```python
from build123d import *

# Parameters (mm, degrees)
SWEEP1_PROFILE_R = 0.425


with BuildPart() as part:
    # Sketch1 → Revolve1 (revolve)
    with BuildSketch(Plane(origin=(0, 0, 0), x_dir=(0, 0, -1), z_dir=(1, 0, 0)), mode=Mode.PRIVATE) as revolve1_sk:
        with BuildLine():
            Line((-2.775, -4.23083487), (-2.775, 0.55))
            Line((-2.775, 0.55), (-2.875, 0.55))
            Line((-2.875, 0.55), (-2.875, 1.55))
            Line((-2.875, 1.55), (-2.775, 1.55))
            Line((-2.775, 1.55), (-2.775, 3.55))
            Line((-2.775, 3.55), (-2.875, 3.55))
            Line((-2.875, 3.55), (-2.875, 4.55))
            Line((-2.875, 4.55), (-2.809348739, 4.55))
            ThreePointArc((-2.809348739, 4.55), (-2.915957278, 4.865659947), (-3.089615901, 5.15))
            ThreePointArc((-3.089615901, 5.15), (-3.34369004, 5.575690752), (-3.487901766, 6.05))
            Line((-3.487901766, 6.05), (-3.589356744, 6.05))
            ThreePointArc((-3.589356744, 6.05), (-3.595964536, 6.714955812), (-3.398660777, 7.35))
            Line((-3.398660777, 7.35), (-3.28656899, 7.35))
            ThreePointArc((-3.28656899, 7.35), (-3.030302783, 7.730047811), (-2.695848299, 8.043494625))
            ThreePointArc((-2.695848299, 8.043494625), (-1.830840994, 8.494415831), (-0.867845076, 8.65))
            Line((-0.867845076, 8.65), (0, 8.65))
            Line((0, 8.65), (0, -8.65))
            Line((0, -8.65), (-0.867845076, -8.65))
            ThreePointArc((-0.867845076, -8.65), (-1.830840994, -8.494415831), (-2.695848299, -8.043494625))
            ThreePointArc((-2.695848299, -8.043494625), (-3.030302783, -7.730047811), (-3.28656899, -7.35))
            Line((-3.28656899, -7.35), (-3.398660777, -7.35))
            ThreePointArc((-3.398660777, -7.35), (-3.595964536, -6.714955812), (-3.589356744, -6.05))
            Line((-3.589356744, -6.05), (-3.487901766, -6.05))
            ThreePointArc((-3.487901766, -6.05), (-3.34369004, -5.575690752), (-3.089615901, -5.15))
            ThreePointArc((-3.089615901, -5.15), (-2.855831908, -4.716593992), (-2.775, -4.23083487))
        make_face()
    revolve(revolve1_sk.sketch.rotate(Axis((0, -8.65, 0), (0, 1, 0)), 180), axis=Axis((0, -8.65, 0), (0, 1, 0)))

    # Sweep1: sweep along a path in Sketch2
    with BuildLine(Plane(origin=(0, 0, 0), x_dir=(0, 0, -1), z_dir=(1, 0, 0))) as sweep1_path:
        Line((-5.08, -14.65), (-5.08, 9.15))
        ThreePointArc((-5.08, 9.15), (-4.347766953, 10.917766953), (-2.58, 11.65))
        Line((-2.58, 11.65), (-2.5, 11.65))
        ThreePointArc((-2.5, 11.65), (-0.732233047, 10.917766953), (0, 9.15))
        Line((0, 9.15), (0, 0))
        Line((0, 0), (0, -14.65))
    # Sweep1 profile (on start of the path) → Sweep1 (sweep)
    with BuildSketch(Plane(origin=(0, -14.65, 5.08), x_dir=(0, 0, 1), z_dir=(0, 1, 0))):
        Circle(SWEEP1_PROFILE_R)
    sweep(path=sweep1_path.line)


solid = part.part
```
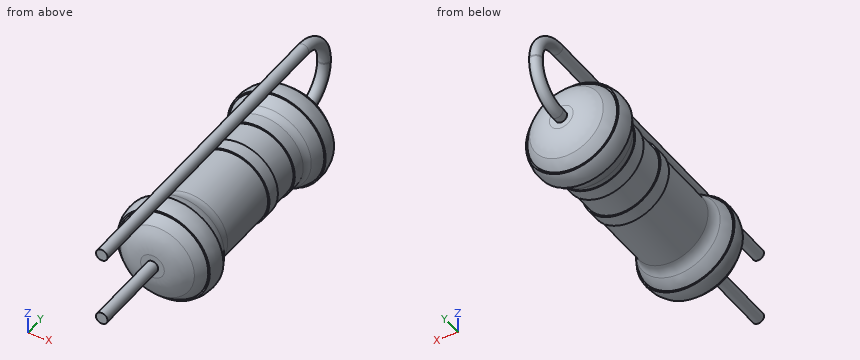
The model under review builds one solid part; all positions refer to its coordinate system, in mm. Coordinates: 2 decimals unless noted, no trailing zeros. Write each loop counter-clockwise with the first axis right and the second up, starting at its lowest first coordinate (ties: lowest second). Pieces come first, ordered by that corner, then holes. Notation, with made-up numbers: (42.5, 37) - (93.5, 37) arc R25 ccw to (93.5, 72) - close; hole circle Ø10 at (57.5, 43.5). An arc over 180 degrees is marked (long way). Answer in a Markdown table with one row per item. Add a question column.
Q1. Clearance check with flat-ended pins moving along their axes: pin 1 (1 mm diameter, centred on x = -2.5, z = 0.5, fed in from +Y); pin 2 (1.5 mm diameter, centred on x = -1, y = 6.5, fed in from -Z); pin 3 (2 mm diameter, centred on x = 1.5, z = -2, fed in from +Y). State where each tip first meets the part, or that it passes through.
Q2. To check wall thickness, follow line 1 along Y through (x, z) = (-1, 0.25); line 2 along Y through (x, z) = (2.75, 1.75); line 3 along Y through (x, z) = (1, -2.75). State the ranges of each line that lie inside material, in increasing order. Write a range as from..to.
Q3. Consider section B-B on y = -12.25. Give the boundary of the cut face in (x, z) (3 decimals).
Q4. Consider section A-A on y = -1.75. Give the boundary of the cut face in (x, z) (3 decimals), then the cut area to 3 significant figures.
Answers below:
| question | item | result |
|---|---|---|
| 1 | pin 1 | y = 8.41 |
| 1 | pin 2 | z = -3.61 |
| 1 | pin 3 | y = 8.58 |
| 2 | line 1 | -8.65..8.65 |
| 2 | line 2 | -7.4..-5.41, 5.41..7.4 |
| 2 | line 3 | -7.84..-4.89, 4.89..7.84 |
| 3 | outline | circle Ø0.85 at (0, 0); circle Ø0.85 at (0, 5.08) |
| 4 | outline | circle Ø5.55 at (0, 0); circle Ø0.85 at (0, 5.08) |
| 4 | area | 24.8 mm² |
